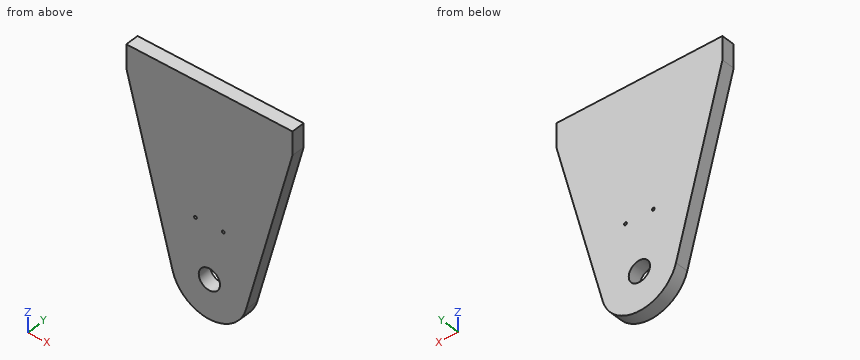
from build123d import *

# Parameters (mm, degrees)
BOSS_EXTRUDE1_DEPTH = 20
SKETCH3_R           = 2.1
SKETCH3_R_2         = 16
CUT_EXTRUDE2_DEPTH  = 20


with BuildPart() as part:
    # Sketch1 → Boss-Extrude1 (new body)
    with BuildSketch(Plane(origin=(0, 0, 0), x_dir=(1, 0, 0), z_dir=(0, 1, 0))):
        with BuildLine():
            Line((-55.118857822, 295.799973098), (-125, 35))
            Line((-125, 35), (-125, 0))
            Line((-125, 0), (125, 0))
            Line((125, 0), (125, 35))
            Line((125, 35), (55.118857822, 295.799973098))
            ThreePointArc((55.118857822, 295.799973098), (0, 338.094160252), (-55.118857822, 295.799973098))
        make_face()
    extrude(amount=BOSS_EXTRUDE1_DEPTH)

    # Sketch3 → Cut-Extrude2 (cut)
    with BuildSketch(Plane(origin=(0, 20, 0), x_dir=(1, 0, 0), z_dir=(0, 1, 0))):
        with Locations(Location((-21, 200, 0), (0, 0, 270))):
            Circle(SKETCH3_R)
        with Locations(Location((21, 200, 0), (0, 0, 90))):
            Circle(SKETCH3_R)
        with Locations(Location((0, 280, 0), (0, 0, 270))):
            Circle(SKETCH3_R_2)
    extrude(amount=-CUT_EXTRUDE2_DEPTH, mode=Mode.SUBTRACT)


solid = part.part
Geometry check sheet. Reference: the model listing, model coordinates, mm. Give positions to 0.01 mm unless a question says otherwise; leave off trailing zeros. Order: outer loops, then holes, each group sorted by start corner. A loop starts at its lowest first (then second) coordinate and runs counter-clockwise, first axis right, second up.
1. Sectioned sample at B-B (x = 0). Record the boundary of the cut face in (y, z).
Completed:
outline: (0, -338.09) - (20, -338.09) - (20, -296) - (0, -296) - close; (0, -264) - (20, -264) - (20, 0) - (0, 0) - close
2. Sectioned sample at A-A (y = 12.75). Record the boundary of the cut face in (x, z).
Completed:
outline: (-125, -35) - (-55.12, -295.8) arc R57.06 ccw to (55.12, -295.8) - (125, -35) - (125, 0) - (-125, 0) - close; hole circle Ø4.2 at (-21, -200); hole circle Ø32 at (0, -280); hole circle Ø4.2 at (21, -200)
3. Scan lines: line 1 (X direction, y = 16.25, z = -200); line 2 (X direction, y = 12, z = -270); line 3 (Z direction, x = 21, y = 6.25). Record each from-to range of solid material in increasing order.
Completed:
line 1: x = -80.79 to -23.1, -18.9 to 18.9, 23.1 to 80.79
line 2: x = -62.03 to -12.49, 12.49 to 62.03
line 3: z = -334.09 to -202.1, -197.9 to 0
4. Sectioned sample at D-D (z = -53). Record the boundary of the cut face in (x, y).
Completed:
outline: (-120.18, 0) - (120.18, 0) - (120.18, 20) - (-120.18, 20) - close
5. Depth check by flat-ended pin: pin 1 (1 mm diameter, centred on y = 2, z = -297.5, fed in from -X); pin 2 (3 mm diameter, centred on y = 8, z = -104, fed in from -X); pin 3 (19 mm diameter, centred on x = 0, z = -280, fed in from -Y); pin 4 (2 mm diameter, centred on y = 6.5, z = -58.5, fed in from +X). Enter the tip coordinate at first touch or a pass-through.
Completed:
pin 1: stops at x = -54.78
pin 2: stops at x = -106.91
pin 3: passes through
pin 4: stops at x = 118.97
6. Sectioned sample at C-C (z = -280). Record the boundary of the cut face in (x, y).
Completed:
outline: (-59.35, 0) - (-16, 0) - (-16, 20) - (-59.35, 20) - close; (16, 0) - (59.35, 0) - (59.35, 20) - (16, 20) - close
